Geometry check sheet. Reference: drawing and pictorial views, mm from the part's lowest x, y, z. A direction names the side the tool comes from. Round coordinates to 2 decimals unless told otherwise and drop trailing zeros. Write each loop counter-clockwise with the first axis right and the second up, starting at its lowest first coordinate (ties: lowest second). Pieces come first, ordered by that corner, then holes.
Item 1: Material ranges on line 1 along X through (y, z) = (34, 4); line 2 along Z through (x, y) = (25, 43); line 3 along X through (y, z) = (18, 2.25), recorded low to high.
Item 2: Section check C-C, the plane y = 19. Record the cut outline in (x, z).
Item 3: Section check D-D, the plane x = 26.5. Record the cut outline in (y, z), plus the area to 3 significant figures.
Item 4: Section check A-A, the plane x = 4. Record the cut outline in (y, z).
Item 5: Set-up check for the marked faces 1, 2 and 3: record each of +Z, -Z, +X, -X, +Y, -Y from which the full face is reachable in a straight line by a thin tool's end or side.
Item 6: Depth check by flat-ended pin: pin 1 (10 mm diameter, centred on x = 35.5, y = 23, fed in from -Z); pin 2 (8 mm diameter, centred on x = 33.5, y = 15.5, fed in from +Z). Enter the tip coordinate at first touch or a pass-through.
Item 7: Section check B-B, the plane z = 4. Record the cut outline in (x, y).
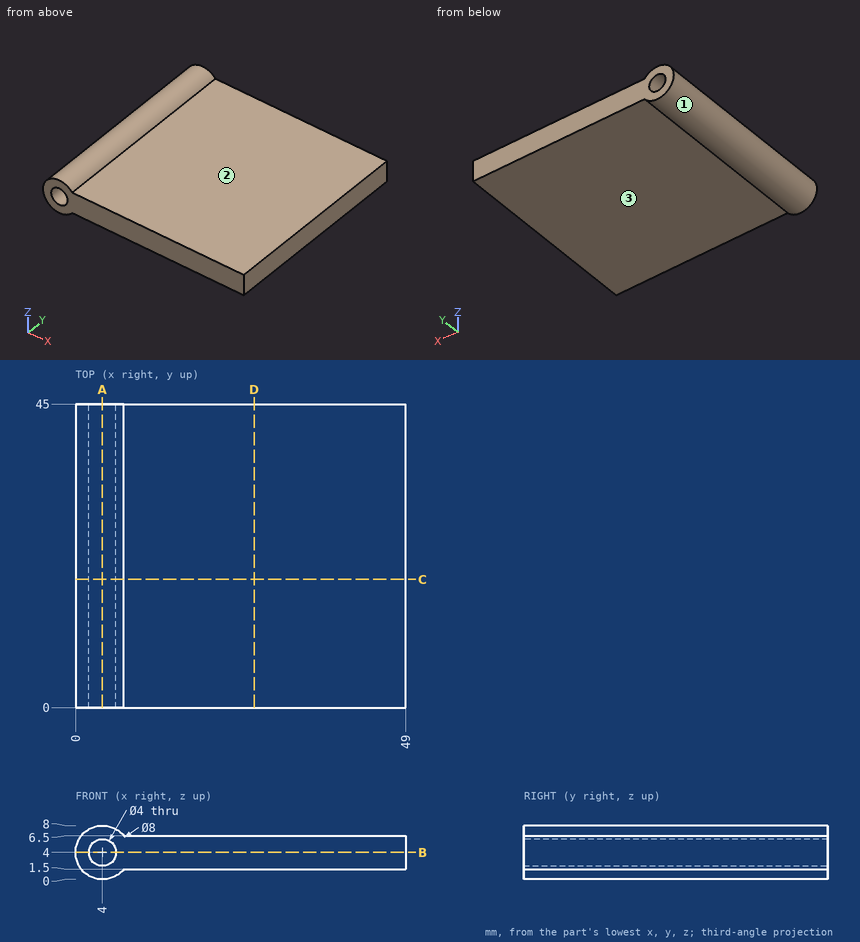
Values found:
1. line 1: x = 0 to 2, 6 to 49
1. line 2: z = 1.5 to 6.5
1. line 3: x = 0.4 to 3.03, 4.97 to 49
2. outline: (7.12, 1.5) - (49, 1.5) - (49, 6.5) - (7.12, 6.5) arc R4 ccw (long way) to start; hole circle Ø4 at (4, 4)
3. outline: (0, 1.5) - (45, 1.5) - (45, 6.5) - (0, 6.5) - close
3. area: 225 mm2
4. outline: (0, 0) - (45, 0) - (45, 2) - (0, 2) - close; (0, 6) - (45, 6) - (45, 8) - (0, 8) - close
5. face 1: +Y, -Y
5. face 2: +Z, +X, +Y, -Y
5. face 3: -Z, +X, +Y, -Y
6. pin 1: stops at z = 1.5
6. pin 2: stops at z = 6.5
7. outline: (0, 0) - (2, 0) - (2, 45) - (0, 45) - close; (6, 0) - (49, 0) - (49, 45) - (6, 45) - close
